from build123d import *

# Parameters (mm, degrees)
SKETCH1_R           = 100.965
BOSS_EXTRUDE1_DEPTH = 386.08
SKETCH2_R           = 51.054
CUT_EXTRUDE1_DEPTH  = 412.637739827
SKETCH3_R           = 22.225
BOSS_EXTRUDE2_DEPTH = 38.1


with BuildPart() as part:
    # Sketch1 → Boss-Extrude1 (new body)
    with BuildSketch(Plane(origin=(0, 0, 0), x_dir=(0, 0, -1), z_dir=(1, 0, 0))):
        Circle(SKETCH1_R)
    extrude(amount=-BOSS_EXTRUDE1_DEPTH)

    # Sketch2 → Cut-Extrude1 (cut, through all)
    with BuildSketch(Plane(origin=(0, 0, 0), x_dir=(0, 0, -1), z_dir=(1, 0, 0))):
        with Locations((0, 19.05)):
            Circle(SKETCH2_R)
    extrude(amount=-CUT_EXTRUDE1_DEPTH, mode=Mode.SUBTRACT)

    # Sketch3 → Boss-Extrude2 (add)
    with BuildSketch(Plane(origin=(0, 0, 0), x_dir=(0, 0, -1), z_dir=(1, 0, 0))):
        with Locations(Location((0, -63.5, 0), (0, 0, 180))):
            Circle(SKETCH3_R)
    extrude(amount=BOSS_EXTRUDE2_DEPTH)


solid = part.part
Work out the finished part from the listing and answer in its coordinate system (mm). Coordinates: 2 decimals unless noted, no trailing zeros. Order: outer loops, then holes, each group sorted by start corner. A loop starts at its lowest first (then second) coordinate and runs counter-clockwise, first axis right, second up. Notation, with made-up numbers: (-19.5, 16.5) - (13.5, 16.5) arc R9 ccw to (13.5, 21.5) - close; hole circle Ø8 at (64.25, 27). An arc over 180 degrees is marked (long way). Put each result on its own line as item: value. Start each with the question number.
1) Find section D-D (y = -51). Give the vertices of the cut face in (x, z), plus the area to 3 significant figures.
2) Find section A-A (z = 0). Give the vertices of the cut face in (x, y) (3 decimals), plus the area to 3 significant figures.
3) Find section C-C (x = -190.5). Give the vertices of the cut face in (y, z) (3 decimals).
4) Flat-ended cylindrical pins translate along their axes: pin 1 (2 mm diameter, centred on x = -306.5, z = -46.5, fed in from -Y); pin 2 (2 mm diameter, centred on x = -29, y = 69.5, fed in from +Z); pin 3 (3 mm diameter, centred on x = -20, y = 21, fed in from +Z). Find the tip coordinate at first contact, or state that the pin passes through.
5) Find the intervals of material crossed by line 1 (Y direction, x = -150, z = 0) (3 decimals); line 2 (X direction, y = 65, z = 47.5); line 3 (Z direction, x = 14, y = -63), in increasing order. Write a range as from..to.
6) Find section B-B (y = 19.05). Give the vertices of the cut face in (x, z).
7) For a pull along Z with two mould halves and no side action, classify faces 1 (the cylindrical face through (-190.337, 34.385, -48.696)), 2 (the flat face through (38.1, -64, 0)), 3 (the cylindrical face through (18.78, -82.24, 11.95)) as released by +Z, released by -Z, zero draft, split by the parting line, or undercut.
Results list:
1. outline: (-386.08, -87.14) - (0, -87.14) - (0, -18.38) - (38.1, -18.38) - (38.1, 18.38) - (0, 18.38) - (0, 87.14) - (-386.08, 87.14) - close
1. area: 68,700 mm^2
2. outline: (-386.08, -100.965) - (0, -100.965) - (0, -85.725) - (38.1, -85.725) - (38.1, -41.275) - (0, -41.275) - (0, -32.004) - (-386.08, -32.004) - close; (-386.08, 70.104) - (0, 70.104) - (0, 100.965) - (-386.08, 100.965) - close
2. area: 40,200 mm^2
3. outline: circle Ø201.93 at (0, 0); hole circle Ø102.108 at (19.05, 0)
4. pin 1: stops at y = -90.13
4. pin 2: stops at z = 74.17
4. pin 3: stops at z = 99.06
5. line 1: y = -100.965..-32.004, 70.104..100.965
5. line 2: x = -386.08..0
5. line 3: z = -22.22..22.22
6. outline: (-386.08, -99.15) - (0, -99.15) - (0, -51.05) - (-386.08, -51.05) - close; (-386.08, 51.05) - (0, 51.05) - (0, 99.15) - (-386.08, 99.15) - close
7. face 1: undercut
7. face 2: zero draft
7. face 3: split by the parting line
